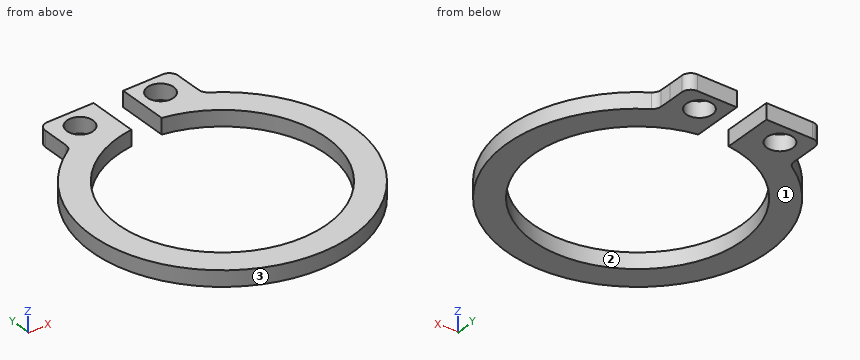
Autodesk Inventor part; units mm, degrees
ref_plane "YZ Plane" through (0, 0, 0) normal (1, 0, 0) x (0, 1, 0)
ref_plane "XZ Plane" through (0, 0, 0) normal (0, 1, 0) x (-1, 0, 0)
ref_plane "XY Plane" through (0, 0, 0) normal (0, 0, 1) x (1, 0, 0)
sketch "Sketch1" plane through (0, 0, 0) normal (0, 0, 1) x (1, 0, 0)
  arc A0 (-4.7345, 8.809) -> (-3.0345, 8.7554) centre (-4.0716, 2.8457) ccw
  line L0 (-0.2689, 9.3429) -> (-0.2689, 11.1409)
  line L1 (-0.7689, 11.6409) -> (-3.0345, 11.6409)
  line L2 (-7.8889, 11.1409) -> (-7.8889, 9.5807)
  circle A1 centre (-1.7689, 10.4919) radius 0.75
  circle A2 centre (-6.3889, 10.4919) radius 0.75
  arc A3 (-8.1191, 9.1598) -> (-0.0285, 9.1626) centre (-4.0716, 2.8457) ccw
  line L3 (-3.0345, 11.6409) -> (-3.0345, 8.7554)
  line L4 (-4.7345, 8.7554) -> (-4.7345, 11.6409)
  line L5 (-4.7345, 11.6409) -> (-7.3889, 11.6409)
  arc A4 (-0.2689, 11.1409) -> (-0.7689, 11.6409) centre (-0.7689, 11.1409) ccw
  arc A5 (-7.3889, 11.6409) -> (-7.8889, 11.1409) centre (-7.3889, 11.1409) ccw
  line L6 (-0.2589, 9.5762) -> (-0.2689, 10.2419)
  arc A6 (-0.2589, 9.5762) -> (-0.0285, 9.1626) centre (0.2411, 9.5837) ccw
  arc A7 (-8.1191, 9.1598) -> (-7.8889, 9.5807) centre (-8.3889, 9.5807) ccw
  point P0 (0, 0)
  point P1 (-7.8889, 9.3015)
  point P2 (-0.2547, 9.3018)
  dimension "d0" = 12
  dimension "d3" = 1.5
  dimension "d4" = 1.5
  dimension "d5" = 7.62
  dimension "d6" = 1.7
  dimension "d7" = 0.75
  dimension "d8" = 0.75
  dimension "d9" = 0.5
  dimension "d12" = 0.5
  dimension "d13" = 0.5
  dimension "d14" = 7.5
extrude "Extrusion1" add sketch "Sketch1" along normal blind 0.9
properties part number "Laasering"
Geometry: final body of the model. Coordinates: model frame, mm. Face numbers are marked on the shaded views. Give positions to 0.01 mm unless a question says otherwise; leave off trailing zeros. Order: outer loops, then holes, each group sorted by start corner. A loop starts at its lowest first (then second) coordinate and runs counter-clockwise, first axis right, second up. Notation, with made-up numbers: (-22.5, 50) -> (-8.5, 50) arc R24 ccw to (-8.5, 84) -> close; hole circle Ø8 at (9, 42). An arc over 180 degrees is marked (long way). Put each result on its own line as item: value.
Q1. Section B-B, the plane x = -6.25. Return loops of the section in (y, z).
Here are the results:
outline: (-4.33, 0) -> (-2.74, 0) -> (-2.74, 0.9) -> (-4.33, 0.9) -> close; (8.44, 0) -> (9.75, 0) -> (9.75, 0.9) -> (8.44, 0.9) -> close; (11.23, 0) -> (11.64, 0) -> (11.64, 0.9) -> (11.23, 0.9) -> close
Q2. Section C-C, the plane x = -0.5. Return loops of the section in (y, z).
Here are the results:
outline: (-3.75, 0) -> (-1.98, 0) -> (-1.98, 0.9) -> (-3.75, 0.9) -> close; (7.67, 0) -> (11.56, 0) -> (11.56, 0.9) -> (7.67, 0.9) -> close
Q3. Material intervals for L1, parallel to X at y = 10, z = 0.1; L2, parallel to Y at x = -7, z = 0.5; L3, parallel to Y at x = -2.25, z = 0.3, sorted ascending.
Here are the results:
L1: x = -7.89 to -6.96, -5.82 to -4.73, -3.03 to -2.34, -1.2 to -0.27
L2: y = -4.06 to -2.39, 8.08 to 10.06, 10.93 to 11.64
L3: y = -4.43 to -2.87, 8.56 to 9.92, 11.07 to 11.64
Q4. Section D-D, the plane z = 0.6. Return loops of the section in (x, y), then the cut area to 3 significant figures.
Here are the results:
outline: (-8.12, 9.16) arc R7.5 ccw (long way) to (-0.03, 9.16) arc R0.5 cw to (-0.26, 9.58) -> (-0.27, 10.24) -> (-0.27, 11.14) arc R0.5 ccw to (-0.77, 11.64) -> (-3.03, 11.64) -> (-3.03, 8.76) arc R6 cw (long way) to (-4.73, 8.81) -> (-4.73, 11.64) -> (-7.39, 11.64) arc R0.5 ccw to (-7.89, 11.14) -> (-7.89, 9.58) arc R0.5 cw to start; hole circle Ø1.5 at (-6.39, 10.49); hole circle Ø1.5 at (-1.77, 10.49)
area: 67.6 mm^2
Q5. Draft query along Y for the marked faces 1, 2 and 3. Return one class per face: released by +Y, released by -Y, zero draft, split by the parting line, or undercut.
Here are the results:
face 1: zero draft
face 2: undercut
face 3: split by the parting line
Q6. Section A-A, the plane y = 7.75. Return loops of the section in (x, z).
Here are the results:
outline: (-9.75, 0) -> (-7.53, 0) -> (-7.53, 0.9) -> (-9.75, 0.9) -> close; (-0.62, 0) -> (1.6, 0) -> (1.6, 0.9) -> (-0.62, 0.9) -> close
